Check sheet for the drawn part. Datum: minimum x, y, z corner. Units: mm. A direction names the side the tool comes from. Give positions to 0.01 mm unless a question says otherwise; leave off trailing zeros. Order: outer loops, then holes, each group sorted by start corner. A loop starts at its lowest first (then second) coordinate and runs counter-clockwise, first axis right, second up.
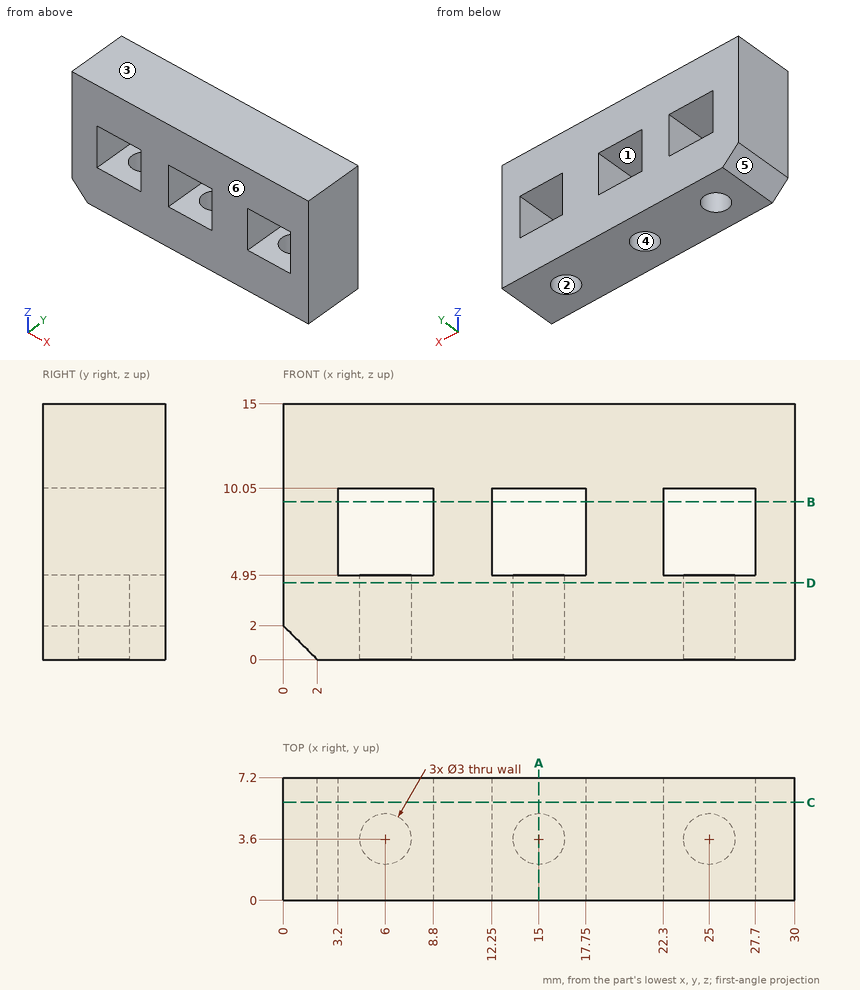
(1) Go/stop test with flat-tipped pins: pin 1 (2 mm diameter, centred on y = 1.5, z = 5.5, fed in from -X); pin 2 (2.5 mm diameter, centred on x = 6, y = 3.6, fed in from -Z). Record where each tip stops, or that it passes through.
Solved:
pin 1: stops at x = 0
pin 2: stops at z = 10.05
(2) Set-up check for the marked faces 1, 2 and 3: record each of +Z, -Z, +X, -X, +Y, -Y from which the full face is reachable in a straight line by a thin tool's end or side.
Solved:
face 1: +Y, -Y
face 2: -Z
face 3: +Z, +X, -X, +Y, -Y
(3) Release check for a two-part mould opening along Y. For the marked faces 4, 5 and 6 record: pulls with the +Y half, pulls with the -Y half, needs draft (parallel to the pull), parting line crosses it, or undercut.
Solved:
face 4: undercut
face 5: needs draft
face 6: pulls with the -Y half
(4) Section check B-B, the plane z = 9.25. Enter the section's corners in (x, y).
Solved:
outline: (0, 0) - (3.2, 0) - (3.2, 7.2) - (0, 7.2) - close; (8.8, 0) - (12.25, 0) - (12.25, 7.2) - (8.8, 7.2) - close; (17.75, 0) - (22.3, 0) - (22.3, 7.2) - (17.75, 7.2) - close; (27.7, 0) - (30, 0) - (30, 7.2) - (27.7, 7.2) - close
(5) Section check C-C, the plane y = 5.75. Enter the section's corners in (x, z), then the cut area to 3 significant figures.
Solved:
outline: (0, 2) - (2, 0) - (30, 0) - (30, 15) - (0, 15) - close; hole (3.2, 4.95) - (8.8, 4.95) - (8.8, 10.05) - (3.2, 10.05) - close; hole (12.25, 4.95) - (17.75, 4.95) - (17.75, 10.05) - (12.25, 10.05) - close; hole (22.3, 4.95) - (27.7, 4.95) - (27.7, 10.05) - (22.3, 10.05) - close
area: 364 mm2
(6) Scan lines: line 1 (X direction, y = 4.25, z = 5.5); line 2 (Y direction, x = 6, z = 2.8); line 3 (Z direction, x = 26, y = 6.5). Record each from-to range of solid material in increasing order.
Solved:
line 1: x = 0 to 3.2, 8.8 to 12.25, 17.75 to 22.3, 27.7 to 30
line 2: y = 0 to 2.1, 5.1 to 7.2
line 3: z = 0 to 4.95, 10.05 to 15
(7) Section check D-D, the plane z = 4.5. Enter the section's corners in (x, y), then the cut area to 3 significant figures.
Solved:
outline: (0, 0) - (30, 0) - (30, 7.2) - (0, 7.2) - close; hole circle Ø3 at (6, 3.6); hole circle Ø3 at (15, 3.6); hole circle Ø3 at (25, 3.6)
area: 195 mm2
(8) Section check A-A, the plane x = 15. Enter the section's corners in (y, z).
Solved:
outline: (0, 0) - (2.1, 0) - (2.1, 4.95) - (0, 4.95) - close; (0, 10.05) - (7.2, 10.05) - (7.2, 15) - (0, 15) - close; (5.1, 0) - (7.2, 0) - (7.2, 4.95) - (5.1, 4.95) - close
